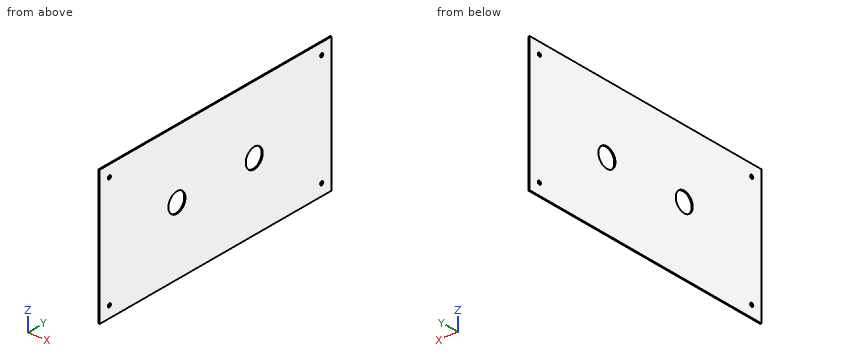
from build123d import *

# Parameters (mm, degrees)
SKETCH1_W                            = 300
SKETCH1_H                            = 150
BOSS_EXTRUDE1_DEPTH                  = 1.3
F_4_0_4_DIAMETER_HOLE1_D             = 4
MIRROR1_AT_THE_SECOND_PLANE_COPY_1_D = 4
F_22_0_22_DIAMETER_HOLE1_D           = 22


with BuildPart() as part:
    # Sketch1 → Boss-Extrude1 (new body)
    with BuildSketch(Plane.YZ):
        Rectangle(SKETCH1_W, SKETCH1_H)
    extrude(amount=BOSS_EXTRUDE1_DEPTH)

    # Ø4.0 (4) Diameter Hole1 (through all)
    with Locations(Plane.YZ.offset(1.3)):
        with Locations((-137.3, 62.3)):
            f_4_0_4_diameter_hole1 = Hole(F_4_0_4_DIAMETER_HOLE1_D / 2)

    # Mirror1: Ø4.0 (4) Diameter Hole1 across plane
    add(f_4_0_4_diameter_hole1.mirror(Plane.ZX), mode=Mode.SUBTRACT)

    # Mirror1 at the second plane: Ø4.0 (4) Diameter Hole1 across plane
    add(f_4_0_4_diameter_hole1.mirror(Plane.XY), mode=Mode.SUBTRACT)

    # Mirror1 at the second plane copy 1 (through all)
    with Locations(Plane(origin=(1.3, 0, 0), x_dir=(0, -1, 0), z_dir=(1, 0, 0))):
        with Locations((-137.3, 62.3)):
            Hole(MIRROR1_AT_THE_SECOND_PLANE_COPY_1_D / 2)

    # Ø22.0 (22) Diameter Hole1 (through all)
    with Locations(Plane.YZ.offset(1.3)):
        with Locations((-50, 0)):
            f_22_0_22_diameter_hole1 = Hole(F_22_0_22_DIAMETER_HOLE1_D / 2)

    # Mirror2: Ø22.0 (22) Diameter Hole1 across plane
    add(f_22_0_22_diameter_hole1.mirror(Plane.ZX), mode=Mode.SUBTRACT)


solid = part.part
For this review, take the finished solid that the model builds, in its own axes (mm). Round coordinates to 2 decimals unless told otherwise and drop trailing zeros. Order: outer loops, then holes, each group sorted by start corner. A loop starts at its lowest first (then second) coordinate and runs counter-clockwise, first axis right, second up. Notation, with made-up numbers: M -23,61 L -14,61 A8 ccw -14,73 Z; hole C -8,48.5 d4. An arc over 180 degrees is marked long. Write each question's results on one line, items separated by ' | '. Start each with the question number.
1. Add section C-C (z = 5). State the section outline as (x, y) points, then the cut area to 3 significant figures.
2. To check wall thickness, follow L1, parallel to Z at x = 0.5, y = 137.3; L2, parallel to Z at x = 0.7, y = -50; L3, parallel to Y at x = 1.05, z = 3. State the ranges of each line that lie inside material, in increasing order. Write a range as [from, to].
3. Add section B-B (x = 0.6). State the section outline as (y, z) points.
4. Add section A-A (y = 50). State the section outline as (x, z) points, then the cut area to 3 significant figures.
5. Add section D-D (y = -47). State the section outline as (x, z) points.
Output values:
1) outline: M 0,-150 L 1.3,-150 L 1.3,-59.8 L 0,-59.8 Z; M 0,-40.2 L 1.3,-40.2 L 1.3,40.2 L 0,40.2 Z; M 0,59.8 L 1.3,59.8 L 1.3,150 L 0,150 Z | area: 339 mm^2
2) L1: [-75, -64.3], [-60.3, 60.3], [64.3, 75] | L2: [-75, -11], [11, 75] | L3: [-150, -60.58], [-39.42, 39.42], [60.58, 150]
3) outline: M -150,-75 L 150,-75 L 150,75 L -150,75 Z; hole C -137.3,-62.3 d4; hole C -137.3,62.3 d4; hole C -50,0 d22; hole C 50,0 d22; hole C 137.3,-62.3 d4; hole C 137.3,62.3 d4
4) outline: M 0,-75 L 1.3,-75 L 1.3,-11 L 0,-11 Z; M 0,11 L 1.3,11 L 1.3,75 L 0,75 Z | area: 166 mm^2
5) outline: M 0,-75 L 1.3,-75 L 1.3,-10.58 L 0,-10.58 Z; M 0,10.58 L 1.3,10.58 L 1.3,75 L 0,75 Z
